CAD build for the part. Positions are in the model's coordinates, mm. Round coordinates to 2 decimals unless told otherwise and drop trailing zeros. Loops run counter-clockwise (first coordinate to the right, second up) from the corner with the lowest first, then second, coordinate; pieces in that order, holes last. Notation, with made-up numbers: (43.5, 30.25) -> (60.5, 30.25) arc R25 cw to (60.5, 57.25) -> close; hole circle Ø7 at (-30.5, 55.25). An arc over 180 degrees is marked (long way). Answer as CSV lines item,"result".
```python
from build123d import *

# Parameters (mm, degrees)
F0_W     = 530
F0_H     = 430
F1_DEPTH = 58
F3_D     = 9
F5_D     = 9
F5_DEPTH = 180
F5_TIP   = 2.7038727856
F7_D     = 9
F7_DEPTH = 180
F7_TIP   = 2.7038727856
F8_W     = 480
F8_H     = 320
F9_DEPTH = 4


# Not quite as in the source:
# - a feature names something its author has since deleted; it is built from what else it names


with BuildPart() as f1:
    # F0 (on Top) → F1 (new body)
    with BuildSketch(Plane.XY):
        with Locations((-265, 215)):
            Rectangle(F0_W, F0_H)
    extrude(amount=F1_DEPTH)

    # F3 (through all)
    with Locations(Plane.XZ):
        with Locations((-450, 33), (-357.5, 33), (-265, 33), (-172.5, 33), (-80, 33)):
            Hole(F3_D / 2)

    # F5
    with Locations(Plane(origin=(-530, 0, 0), x_dir=(0, -1, 0), z_dir=(-1, 0, 0))):
        with Locations((-330, 33)):
            Hole(F5_D / 2, depth=F5_DEPTH)
            with Locations((0, 0, -(F5_DEPTH + F5_TIP / 2))):  # 118° drill point
                Cone(0, F5_D / 2, F5_TIP, mode=Mode.SUBTRACT)

    # F7
    with Locations(Plane.YZ):
        with Locations((330, 33)):
            Hole(F7_D / 2, depth=F7_DEPTH)
            with Locations((0, 0, -(F7_DEPTH + F7_TIP / 2))):  # 118° drill point
                Cone(0, F7_D / 2, F7_TIP, mode=Mode.SUBTRACT)

    # F8 (on face) → F9 (cut)
    with BuildSketch(Plane.XY.offset(58)):
        with Locations((-265, 215)):
            Rectangle(F8_W, F8_H)
    extrude(amount=-F9_DEPTH, mode=Mode.SUBTRACT)


solid = f1.part
```
Q1. Drop flat-ended pins along their axis: pin 1 Ø6 at (x, z) = (-264, 34.5) entering from -Y; pin 2 Ø5.5 at (y, z) = (330, 33) entering from -X; pin 3 Ø7 at (y, z) = (330, 33) entering from +X; pin 4 Ø8 at (y, z) = (330, 33) entering from -X. Give the stop position or say it passes through.
Results:
pin 1,"y = 0"
pin 2,"x = -348.95"
pin 3,"x = -180.6"
pin 4,"x = -349.7"
Q2. Slice it at A-A, the plane y = 91. Give the cut face in (x, z).
Results:
outline,"(-530, 0) -> (0, 0) -> (0, 58) -> (-25, 58) -> (-25, 54) -> (-505, 54) -> (-505, 58) -> (-530, 58) -> close; hole circle Ø9 at (-450, 33); hole circle Ø9 at (-357.5, 33); hole circle Ø9 at (-265, 33); hole circle Ø9 at (-172.5, 33); hole circle Ø9 at (-80, 33)"
Q3. Probe L1, parallel to X at y = 192.5, z = 54.5; L2, parallel to Z at x = -80, y = 381; L3, parallel to Y at x = -496.5, z = 33. List the from-to ranges inside material, lowest first. Write a range as [from, to].
Results:
L1,"[-530, -505], [-25, 0]"
L2,"[0, 28.5], [37.5, 58]"
L3,"[0, 325.5], [334.5, 430]"
Q4. Slice it at B-B, the plane x = -208. Give the cut face in (y, z).
Results:
outline,"(0, 0) -> (430, 0) -> (430, 58) -> (375, 58) -> (375, 54) -> (55, 54) -> (55, 58) -> (0, 58) -> close"
Q5. Two-plate mould, pull along Y, no slides. Class faces 1 (the flat face through (-269, 430, 29)), 2 (the flat face through (0, 212, 29)), 3 (the flat face through (-268, 217, 54)): pulls with the +Y half, pulls with the -Y half, needs draft (parallel to the pull), parting line crosses it, or undercut.
Results:
face 1,"pulls with the +Y half"
face 2,"needs draft"
face 3,"undercut"
